For this review, take the finished solid that the model builds, in its own axes (mm). A direction names the side the tool comes from. Coordinates: 2 decimals unless noted, no trailing zeros. One line per item, written item: value. Start each with the question number.
(1) Mouldability with a two-part tool opening along X and no side actions: class faces 1 (the flat face through (22.5, 0, 31)), 2 (the flat face through (-22.5, 0, 31)), 3 (the flat face through (-21.5, 0, 31)), 4 (the flat face through (0, -22.5, 31)) as released by +X, released by -X, zero draft, split by the parting line, or undercut.
(2) To check wall thickness, follow line 1 along X through (y, z) = (-4.5, 30); line 2 along X through (y, z) = (-0.5, 21.5) (3 decimals); line 3 along Z through (x, y) = (-11, 4.5). State the ranges of each line that lie inside material, in increasing order.
(3) For faces 5 (the flat face through (0, 22.5, 31)), 6 (the flat face through (0, 0, 0)), list the 3-axis set-ups (+Z, -Z, +X, -X, +Y, -Y) from which the entire face can be reached by the end or side of a thin tool; tool diameter is ignored.
(4) Clearance check with flat-ended pins moving along their axes: pin 1 (0.8 mm diameter, centred on y = 1, z = -0.5, fed in from -X); pin 2 (4 mm diameter, centred on x = -5, z = 19, fed in from +Y); pin 3 (3 mm diameter, centred on y = 2.5, z = 19, fed in from -X) (3 decimals); pin 4 (6 mm diameter, centred on x = -16, y = -1, fed in from -Z). State where each tip first meets the part, or that it passes through.
```python
from build123d import *

# Parameters (mm, degrees)
F0_W     = 28
F0_H     = 28
F7_DEPTH = 1
F8_DEPTH = 1.5


with BuildPart() as f3:
    # F2 (on offset) → F3 section 0
    with BuildSketch(Plane.XY.offset(30)):
        Polygon((22.5, -22.5), (21.5, -21.5), (-21.5, -21.5), (-22.5, -22.5), align=None)
    # F0 (on Top) → F3 section 1
    with BuildSketch(Plane.XY):
        Polygon((15, -15), (14, -14), (-14, -14), (-15, -15), align=None)
    loft()

    # F0 (on Top) → F4 section 0
    with BuildSketch(Plane.XY):
        Polygon((14, 14), (14, -14), (15, -15), (15, 15), align=None)
    # F2 (on offset) → F4 section 1
    with BuildSketch(Plane.XY.offset(30)):
        Polygon((21.5, 21.5), (21.5, -21.5), (22.5, -22.5), (22.5, 22.5), align=None)
    loft()

    # F0 (on Top) → F5 section 0
    with BuildSketch(Plane.XY):
        Polygon((-14, 14), (14, 14), (15, 15), (-15, 15), align=None)
    # F2 (on offset) → F5 section 1
    with BuildSketch(Plane.XY.offset(30)):
        Polygon((-21.5, 21.5), (21.5, 21.5), (22.5, 22.5), (-22.5, 22.5), align=None)
    loft()

    # F0 (on Top) → F6 section 0
    with BuildSketch(Plane.XY):
        Polygon((-15, -15), (-14, -14), (-14, 14), (-15, 15), align=None)
    # F2 (on offset) → F6 section 1
    with BuildSketch(Plane.XY.offset(30)):
        Polygon((-22.5, -22.5), (-21.5, -21.5), (-21.5, 21.5), (-22.5, 22.5), align=None)
    loft()

    # F0 (on Top) → F7 (join)
    with BuildSketch(Plane.XY):
        Polygon((-14, 14), (14, 14), (15, 15), (-15, 15), align=None)
        Polygon((-15, -15), (-14, -14), (-14, 14), (-15, 15), align=None)
        Polygon((15, -15), (14, -14), (-14, -14), (-15, -15), align=None)
        Polygon((14, 14), (14, -14), (15, -15), (15, 15), align=None)
        Rectangle(F0_W, F0_H)
    extrude(amount=-F7_DEPTH)

    # F2 (on offset) → F8 (join)
    with BuildSketch(Plane.XY.offset(30)):
        Polygon((22.5, -22.5), (21.5, -21.5), (-21.5, -21.5), (-22.5, -22.5), align=None)
        Polygon((21.5, 21.5), (21.5, -21.5), (22.5, -22.5), (22.5, 22.5), align=None)
        Polygon((-21.5, 21.5), (21.5, 21.5), (22.5, 22.5), (-22.5, 22.5), align=None)
        Polygon((-22.5, -22.5), (-21.5, -21.5), (-21.5, 21.5), (-22.5, 22.5), align=None)
    extrude(amount=F8_DEPTH)


solid = f3.part
```
Geometry check:
1. face 1: released by +X
1. face 2: released by -X
1. face 3: undercut
1. face 4: zero draft
2. line 1: x = -22.5 to -21.5, 21.5 to 22.5
2. line 2: x = -20.375 to -19.375, 19.375 to 20.375
2. line 3: z = -1 to 0
3. face 5: +Z, -Z, +X, -X, +Y
3. face 6: +Z
4. pin 1: stops at x = -15
4. pin 2: stops at y = 20.25
4. pin 3: stops at x = -20.125
4. pin 4: stops at z = -1
